Design review of the part built by this model. Coordinates are the model's own, in mm. A direction names the side the tool comes from. Coordinates: 2 decimals unless noted, no trailing zeros. Write each loop counter-clockwise with the first axis right and the second up, starting at its lowest first coordinate (ties: lowest second). Pieces come first, ordered by that corner, then holes.
Q1. For probe 1 along Y at (x, z) = (0, 2.5); probe 2 along Z at (x, y) = (3, 4.5); probe 3 along Y at (x, z) = (0, 3.25), list the stretches that pass through material, from the lowest coordinate up.
Q2. Machinability: for faces 4 (the flat face through (1, 2, 8.5)), 5 (the cylindrical face through (-28.283, 0.541, 1.479)), which of the approach directions +Z, -Z, +X, -X, +Y, -Y give a long, thin tool a straight path to every point of the face, cutting with its end or side? Answer none if there is none.
Q3. Take a section at C-C (z = 6.25). Give the boundary of the cut face in (x, y).
Q4. Take a section at B-B (z = 9.25). Give the boundary of the cut face in (x, y), and give its area (3 significant figures).
Q5. Mouldability with a two-part tool opening along X and no side actions: class faces 1 (the cylindrical face through (-14.995, -1.057, 1.479)), 2 (the flat face through (3, 1, 11)), 3 (the cylindrical face through (-0.878, -3.954, 6.944)) as pulls with the +X half, pulls with the -X half, needs draft (parallel to the pull), parting line crosses it, or undercut.
Q6. Insertion check: pin 1 (1 mm diameter, centred on x = -24, z = 4.5, fed in from -Y); pin 2 (2 mm diameter, centred on x = -21.5, z = 1.5, fed in from +Y); pin 3 (1 mm diameter, centred on x = 1, z = 7, fed in from +Y); pin 4 (2 mm diameter, centred on x = -0.5, z = 9.5, fed in from -Y). Each pin has a flat end and moves straight along its axis. Give the tip position at first contact, or say it passes through.
Q7. Take a section at D-D (x = -25). Give the boundary of the cut face in (y, z), and give its area (3 significant figures).
Q8. Take a section at A-A (x = 0). Give the boundary of the cut face in (y, z).
```python
from build123d import *

# Parameters (mm, degrees)
SKETCH1_R               = 4.05
SKETCH1_R_2             = 1.8
BOSS_EXTRUDE1_DEPTH     = 3
SKETCH1_2_R             = 4.05
BOSS_EXTRUDE2_DEPTH     = 11
FILLET1_R               = 5
SKETCH2_R               = 1.85
CUT_EXTRUDE1_DEPTH      = 37.235341864
CUT_EXTRUDE2_DEPTH      = 2.5
CUT_EXTRUDE3_DEPTH      = 36.440090293
CUT_EXTRUDE3_DEPTH_BACK = 36.440090293
FILLET2_R               = 8


with BuildPart() as part:
    # Sketch1 → Boss-Extrude1 (new body)
    with BuildSketch(Plane.XY):
        with BuildLine():
            Line((-7, 6), (-30.343961021, 3.985183912))
            ThreePointArc((-30.343961021, 3.985183912), (-34, 0), (-30.343961021, -3.985183912))
            Line((-30.343961021, -3.985183912), (-7, -6))
            Line((-7, -6), (7, -6))
            Line((7, -6), (7, 6))
            Line((7, 6), (-7, 6))
        make_face()
        Circle(SKETCH1_R, mode=Mode.SUBTRACT)
        with Locations((-30, 0)):
            Circle(SKETCH1_R_2, mode=Mode.SUBTRACT)
    extrude(amount=BOSS_EXTRUDE1_DEPTH)

    # Sketch1<2> → Boss-Extrude2 (add)
    with BuildSketch(Plane.XY):
        Circle(SKETCH1_2_R)
    extrude(amount=BOSS_EXTRUDE2_DEPTH)

    # Fillet1
    fillet1_edges = [part.edges().sort_by_distance(p)[0] for p in [
        (7, 6, 1.5),
        (7, -6, 1.5),
    ]]
    fillet(fillet1_edges, radius=FILLET1_R)

    # Sketch2 → Cut-Extrude1 (cut, through all)
    with BuildSketch(Plane(origin=(0, 0, 0), x_dir=(-1, 0, 0), z_dir=(0, 0, -1))):
        Circle(SKETCH2_R)
    extrude(amount=-CUT_EXTRUDE1_DEPTH, mode=Mode.SUBTRACT)

    # Sketch3 → Cut-Extrude2 (cut)
    with BuildSketch(Plane.XY.offset(11)):
        Polygon((1.558845727, 2.7), (-1.558845727, 2.7), (-3.117691454, 0), (-1.558845727, -2.7), (1.558845727, -2.7), (3.117691454, 0), align=None)
    extrude(amount=-CUT_EXTRUDE2_DEPTH, mode=Mode.SUBTRACT)

    # Sketch5 → Cut-Extrude3 (cut, two sides: drawn at the far end of the back side and taken through both)
    with BuildSketch(Plane.XY.offset(3).offset(-CUT_EXTRUDE3_DEPTH_BACK)):
        with BuildLine():
            Line((-27.410855082, -4.238340137), (-7, -6))
            Line((-7, -6), (-3.277962863, -6))
            Line((-3.277962863, -6), (-3.271243445, -6))
            ThreePointArc((-3.271243445, -6), (-15.044311785, -1.053046052), (-27.410855082, -4.238340137))
        make_face()
    extrude(amount=CUT_EXTRUDE3_DEPTH + CUT_EXTRUDE3_DEPTH_BACK, mode=Mode.SUBTRACT)

    # Fillet2
    fillet2_edges = [part.edges().sort_by_distance(p)[0] for p in [
        (-27.410855082, -4.238340137, 1.5),
        (-3.271243445, -6, 1.5),
    ]]
    fillet(fillet2_edges, radius=FILLET2_R)


solid = part.part
```
Response:
1. probe 1: y = -6 to -1.85, 1.85 to 6
1. probe 2: z = 0 to 3
1. probe 3: y = -4.05 to -1.85, 1.85 to 4.05
2. face 4: +Z
2. face 5: +Z, -Z
3. outline: circle Ø8.1 at (0, 0); hole circle Ø3.7 at (0, 0)
4. outline: circle Ø8.1 at (0, 0); hole (-3.12, 0) - (-1.56, -2.7) - (1.56, -2.7) - (3.12, 0) - (1.56, 2.7) - (-1.56, 2.7) - close
4. area: 26.3 mm2
5. face 1: undercut
5. face 2: needs draft
5. face 3: parting line crosses it
6. pin 1: passes through
6. pin 2: stops at y = 4.83
6. pin 3: stops at y = 4.02
6. pin 4: stops at y = -4.05
7. outline: (-2.9, 0) - (4.45, 0) - (4.45, 3) - (-2.9, 3) - close
7. area: 22.0 mm2
8. outline: (-6, 0) - (-1.85, 0) - (-1.85, 8.5) - (-2.7, 8.5) - (-2.7, 11) - (-4.05, 11) - (-4.05, 3) - (-6, 3) - close; (1.85, 0) - (6, 0) - (6, 3) - (4.05, 3) - (4.05, 11) - (2.7, 11) - (2.7, 8.5) - (1.85, 8.5) - close
